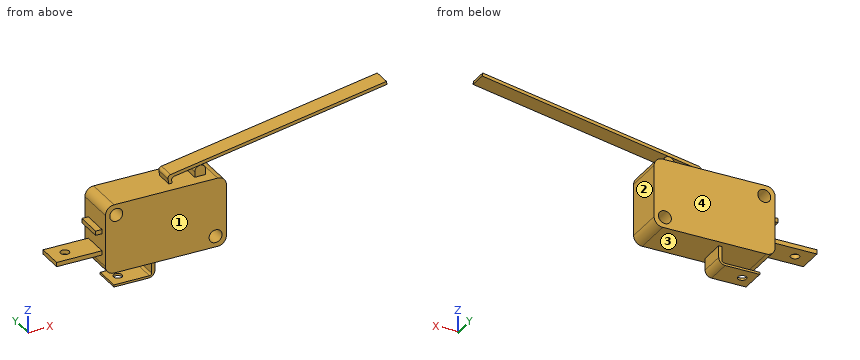
```python
from build123d import *

# Parameters (mm, degrees)
F0_R           = 1.5
F1_DEPTH       = 4.5
F0_W           = 1.5
F0_H           = 1
F0_W_2         = 10.5
F2_DEPTH       = 3
F3_DEPTH       = 2
F4_DEPTH       = 4.5
F5_DEPTH       = 3
F6_DEPTH       = 2
F9_D           = 2
F9_DEPTH       = 1
F9_TIP         = 0.600860619
F9_ON_F8_D     = 2
F9_ON_F8_DEPTH = 1
F9_ON_F8_TIP   = 0.600860619


with BuildPart() as f1:
    # F0 (on Front) → F1 (new body)
    with BuildSketch(Plane.XZ):
        with BuildLine():
            Line((16.1163130835, 15.3639883176), (2.1163130835, 15.3639883176))
            ThreePointArc((2.1163130835, 15.3639883176), (0.7020995211, 14.77820188), (0.1163130835, 13.3639883176))
            Line((0.1163130835, 13.3639883176), (0.1163130835, 9.3639883176))
            Line((0.1163130835, 9.3639883176), (0.1163130835, 8.3639883176))
            Line((0.1163130835, 8.3639883176), (0.1163130835, 4.3639883176))
            Line((0.1163130835, 4.3639883176), (0.1163130835, 3.3639883176))
            Line((0.1163130835, 3.3639883176), (0.1163130835, 1.3639883176))
            ThreePointArc((0.1163130835, 1.3639883176), (0.7020995211, -0.0502252447), (2.1163130835, -0.6360116824))
            Line((2.1163130835, -0.6360116824), (11.6163130835, -0.6360116824))
            Line((11.6163130835, -0.6360116824), (12.3663130835, -0.6360116824))
            Line((12.3663130835, -0.6360116824), (26.1163130835, -0.6360116824))
            ThreePointArc((26.1163130835, -0.6360116824), (27.5305266458, -0.0502252447), (28.1163130835, 1.3639883176))
            Line((28.1163130835, 1.3639883176), (28.1163130835, 13.3639883176))
            ThreePointArc((28.1163130835, 13.3639883176), (27.5305266458, 14.77820188), (26.1163130835, 15.3639883176))
            Line((26.1163130835, 15.3639883176), (24.6163130835, 15.3639883176))
            Line((24.6163130835, 15.3639883176), (23.3663130835, 15.3639883176))
            Line((23.3663130835, 15.3639883176), (22.1163130835, 15.3639883176))
            Line((22.1163130835, 15.3639883176), (16.8778830424, 15.3639883176))
            Line((16.8778830424, 15.3639883176), (16.1163130835, 15.3639883176))
        make_face()
        with Locations((25.6163130835, 1.8639883176)):
            Circle(F0_R, mode=Mode.SUBTRACT)
        with Locations((2.6163130835, 12.8639883176)):
            Circle(F0_R, mode=Mode.SUBTRACT)
    extrude(amount=F1_DEPTH)

    # F0 (on Front) → F2 (join)
    with BuildSketch(Plane.XZ):
        with Locations((-0.6336869165, 8.8639883176)):
            Rectangle(F0_W, F0_H)
        with Locations((-5.1336869165, 3.8639883176)):
            Rectangle(F0_W_2, F0_H)
        with BuildLine():
            Line((12.3663130835, -0.6360116824), (11.6163130835, -0.6360116824))
            Line((11.6163130835, -0.6360116824), (11.6163130835, -3.8694406524))
            ThreePointArc((11.6163130835, -3.8694406524), (11.4698664741, -4.222994043), (11.1163130835, -4.3694406524))
            Line((11.1163130835, -4.3694406524), (2.8663130835, -4.3694406524))
            Line((2.8663130835, -4.3694406524), (2.8663130835, -4.8694406524))
            Line((2.8663130835, -4.8694406524), (10.8663130835, -4.8694406524))
            ThreePointArc((10.8663130835, -4.8694406524), (11.9269732552, -4.4301008242), (12.3663130835, -3.3694406524))
            Line((12.3663130835, -3.3694406524), (12.3663130835, -0.6360116824))
        make_face()
    extrude(amount=F2_DEPTH)

    # F0 (on Front) → F3 (join)
    with BuildSketch(Plane.XZ):
        with BuildLine():
            Line((15.8992528614, 16.5949980089), (16.1163130835, 15.3639883176))
            Line((16.1163130835, 15.3639883176), (16.8778830424, 15.3639883176))
            Line((16.8778830424, 15.3639883176), (16.7680948094, 15.9866283274))
            ThreePointArc((16.7680948094, 15.9866283274), (16.8923365909, 16.5470467879), (17.3764644909, 16.8554702754))
            Line((17.3764644909, 16.8554702754), (66.6168521415, 25.5378791587))
            Line((66.6168521415, 25.5378791587), (66.4866160083, 26.2764849735))
            Line((66.4866160083, 26.2764849735), (16.5076225429, 17.4638399569))
            ThreePointArc((16.5076225429, 17.4638399569), (16.0234946429, 17.1554164694), (15.8992528614, 16.5949980089))
        make_face()
        with BuildLine():
            ThreePointArc((24.6163130835, 16.6139883176), (24.25019656, 15.7301048411), (23.3663130835, 15.3639883176))
            Line((23.3663130835, 15.3639883176), (24.6163130835, 15.3639883176))
            Line((24.6163130835, 15.3639883176), (24.6163130835, 16.6139883176))
        make_face()
        with BuildLine():
            Line((22.1163130835, 16.6139883176), (22.1163130835, 15.3639883176))
            Line((22.1163130835, 15.3639883176), (23.3663130835, 15.3639883176))
            ThreePointArc((23.3663130835, 15.3639883176), (22.482429607, 15.7301048411), (22.1163130835, 16.6139883176))
        make_face()
        with BuildLine():
            ThreePointArc((22.1163130835, 16.6139883176), (22.482429607, 15.7301048411), (23.3663130835, 15.3639883176))
            ThreePointArc((23.3663130835, 15.3639883176), (24.25019656, 15.7301048411), (24.6163130835, 16.6139883176))
            Line((24.6163130835, 16.6139883176), (22.1163130835, 16.6139883176))
        make_face()
        with BuildLine():
            ThreePointArc((24.6163130835, 16.6139883176), (23.3663130835, 17.8639883176), (22.1163130835, 16.6139883176))
            Line((22.1163130835, 16.6139883176), (24.6163130835, 16.6139883176))
        make_face()
    extrude(amount=F3_DEPTH)

    # F0 (on Front) → F4 (join)
    with BuildSketch(Plane.XZ):
        with BuildLine():
            Line((16.1163130835, 15.3639883176), (2.1163130835, 15.3639883176))
            ThreePointArc((2.1163130835, 15.3639883176), (0.7020995211, 14.77820188), (0.1163130835, 13.3639883176))
            Line((0.1163130835, 13.3639883176), (0.1163130835, 9.3639883176))
            Line((0.1163130835, 9.3639883176), (0.1163130835, 8.3639883176))
            Line((0.1163130835, 8.3639883176), (0.1163130835, 4.3639883176))
            Line((0.1163130835, 4.3639883176), (0.1163130835, 3.3639883176))
            Line((0.1163130835, 3.3639883176), (0.1163130835, 1.3639883176))
            ThreePointArc((0.1163130835, 1.3639883176), (0.7020995211, -0.0502252447), (2.1163130835, -0.6360116824))
            Line((2.1163130835, -0.6360116824), (11.6163130835, -0.6360116824))
            Line((11.6163130835, -0.6360116824), (12.3663130835, -0.6360116824))
            Line((12.3663130835, -0.6360116824), (26.1163130835, -0.6360116824))
            ThreePointArc((26.1163130835, -0.6360116824), (27.5305266458, -0.0502252447), (28.1163130835, 1.3639883176))
            Line((28.1163130835, 1.3639883176), (28.1163130835, 13.3639883176))
            ThreePointArc((28.1163130835, 13.3639883176), (27.5305266458, 14.77820188), (26.1163130835, 15.3639883176))
            Line((26.1163130835, 15.3639883176), (24.6163130835, 15.3639883176))
            Line((24.6163130835, 15.3639883176), (23.3663130835, 15.3639883176))
            Line((23.3663130835, 15.3639883176), (22.1163130835, 15.3639883176))
            Line((22.1163130835, 15.3639883176), (16.8778830424, 15.3639883176))
            Line((16.8778830424, 15.3639883176), (16.1163130835, 15.3639883176))
        make_face()
        with Locations((25.6163130835, 1.8639883176)):
            Circle(F0_R, mode=Mode.SUBTRACT)
        with Locations((2.6163130835, 12.8639883176)):
            Circle(F0_R, mode=Mode.SUBTRACT)
    extrude(amount=-F4_DEPTH)

    # F0 (on Front) → F5 (join)
    with BuildSketch(Plane.XZ):
        with Locations((-0.6336869165, 8.8639883176)):
            Rectangle(F0_W, F0_H)
        with Locations((-5.1336869165, 3.8639883176)):
            Rectangle(F0_W_2, F0_H)
        with BuildLine():
            Line((12.3663130835, -0.6360116824), (11.6163130835, -0.6360116824))
            Line((11.6163130835, -0.6360116824), (11.6163130835, -3.8694406524))
            ThreePointArc((11.6163130835, -3.8694406524), (11.4698664741, -4.222994043), (11.1163130835, -4.3694406524))
            Line((11.1163130835, -4.3694406524), (2.8663130835, -4.3694406524))
            Line((2.8663130835, -4.3694406524), (2.8663130835, -4.8694406524))
            Line((2.8663130835, -4.8694406524), (10.8663130835, -4.8694406524))
            ThreePointArc((10.8663130835, -4.8694406524), (11.9269732552, -4.4301008242), (12.3663130835, -3.3694406524))
            Line((12.3663130835, -3.3694406524), (12.3663130835, -0.6360116824))
        make_face()
    extrude(amount=-F5_DEPTH)

    # F0 (on Front) → F6 (join)
    with BuildSketch(Plane.XZ):
        with BuildLine():
            ThreePointArc((24.6163130835, 16.6139883176), (23.3663130835, 17.8639883176), (22.1163130835, 16.6139883176))
            Line((22.1163130835, 16.6139883176), (24.6163130835, 16.6139883176))
        make_face()
        with BuildLine():
            ThreePointArc((22.1163130835, 16.6139883176), (22.482429607, 15.7301048411), (23.3663130835, 15.3639883176))
            ThreePointArc((23.3663130835, 15.3639883176), (24.25019656, 15.7301048411), (24.6163130835, 16.6139883176))
            Line((24.6163130835, 16.6139883176), (22.1163130835, 16.6139883176))
        make_face()
        with BuildLine():
            ThreePointArc((24.6163130835, 16.6139883176), (24.25019656, 15.7301048411), (23.3663130835, 15.3639883176))
            Line((23.3663130835, 15.3639883176), (24.6163130835, 15.3639883176))
            Line((24.6163130835, 15.3639883176), (24.6163130835, 16.6139883176))
        make_face()
        with BuildLine():
            Line((22.1163130835, 16.6139883176), (22.1163130835, 15.3639883176))
            Line((22.1163130835, 15.3639883176), (23.3663130835, 15.3639883176))
            ThreePointArc((23.3663130835, 15.3639883176), (22.482429607, 15.7301048411), (22.1163130835, 16.6139883176))
        make_face()
        with BuildLine():
            Line((15.8992528614, 16.5949980089), (16.1163130835, 15.3639883176))
            Line((16.1163130835, 15.3639883176), (16.8778830424, 15.3639883176))
            Line((16.8778830424, 15.3639883176), (16.7680948094, 15.9866283274))
            ThreePointArc((16.7680948094, 15.9866283274), (16.8923365909, 16.5470467879), (17.3764644909, 16.8554702754))
            Line((17.3764644909, 16.8554702754), (66.6168521415, 25.5378791587))
            Line((66.6168521415, 25.5378791587), (66.4866160083, 26.2764849735))
            Line((66.4866160083, 26.2764849735), (16.5076225429, 17.4638399569))
            ThreePointArc((16.5076225429, 17.4638399569), (16.0234946429, 17.1554164694), (15.8992528614, 16.5949980089))
        make_face()
    extrude(amount=-F6_DEPTH)

    # F9
    with Locations(Plane(origin=(0, 0, -4.8694406524), x_dir=(1, 0, 0), z_dir=(0, 0, -1))):
        with Locations((5.3663130835, 0)):
            Hole(F9_D / 2, depth=F9_DEPTH)
            with Locations((0, 0, -(F9_DEPTH + F9_TIP / 2))):  # 118° drill point
                Cone(0, F9_D / 2, F9_TIP, mode=Mode.SUBTRACT)

    # F9 on F8
    with Locations(Plane(origin=(0, 0, 3.3639883176), x_dir=(1, 0, 0), z_dir=(0, 0, -1))):
        with Locations((-6.8836869165, 0)):
            Hole(F9_ON_F8_D / 2, depth=F9_ON_F8_DEPTH)
            with Locations((0, 0, -(F9_ON_F8_DEPTH + F9_ON_F8_TIP / 2))):  # 118° drill point
                Cone(0, F9_ON_F8_D / 2, F9_ON_F8_TIP, mode=Mode.SUBTRACT)


solid = f1.part
```
Check sheet for the modelled part. Datum: model origin and axes. Units: mm. Face numbers are marked on the shaded views. A direction names the side the tool comes from. Give positions to 0.01 mm unless a question says otherwise; leave off trailing zeros. Order: outer loops, then holes, each group sorted by start corner. A loop starts at its lowest first (then second) coordinate and runs counter-clockwise, first axis right, second up. Notation, with made-up numbers: (62.25, 26.5) -> (81.25, 26.5) arc R34 ccw to (81.25, 62.5) -> close; hole circle Ø4 at (1, 84). An arc over 180 degrees is marked (long way). Use CSV: the item, a comma, the result in double quotes. Start each with the question number.
1) Go/stop test with flat-tipped pins: P1, Ø5, axis at y = 1, z = 12, coming from the +X side; P2, Ø2, axis at x = 23.5, z = 17, coming from the +Y side; P3, Ø0.8, axis at x = 23.5, z = 16.5, coming from the -Y side; P4, Ø5, axis at x = 32.5, z = 16, coming from the -Y side. Record where each tip stops, or that it passes through.
2) Sectioned sample at C-C, the plane x = 19. Record the boundary of the cut face in (y, z).
3) Sectioned sample at B-B, the plane y = 0. Give the number of separate pieces and of enclosed holes in the cut face, plus the area to 3 significant figures.
4) Set-up check for the marked faces 1 and 2: record each of +Z, -Z, +X, -X, +Y, -Y from which the full face is reachable in a straight line by a thin tool's end or side.
5) Sectioned sample at A-A, the plane x = 8. Record the boundary of the cut face in (y, z).
6) Sectioned sample at D-D, the plane x = 47.5. Record the boundary of the cut face in (y, z), plus the area to 3 significant figures.
7) Material ranges on line 1 (Z direction, x = 0, y = 1); line 2 (X direction, y = -3, z = 6); line 3 (Z direction, x = 7, y = -2.5), recorded low to high. Write a range as from..to.
8) Mould release check, pull along Z, two halves, no side actions. Record for the marked faces 3 and 4: released by +Z, released by -Z, zero draft, split by the parting line, or undercut.
Recorded:
1,P1,"x = 28.12"
1,P2,"y = 2"
1,P3,"y = -2"
1,P4,"through"
2,outline,"(-4.5, -0.64) -> (4.5, -0.64) -> (4.5, 15.36) -> (-4.5, 15.36) -> close; (-2, 17.14) -> (2, 17.14) -> (2, 17.9) -> (-2, 17.9) -> close"
3,separate pieces,"3"
3,enclosed holes,"2"
3,area,"492 mm2"
4,face 1,"+Z, -Z, +X, -X, -Y"
4,face 2,"-Z, +X, +Y, -Y"
5,outline,"(-4.5, -0.64) -> (4.5, -0.64) -> (4.5, 15.36) -> (-4.5, 15.36) -> close; (-3, -4.87) -> (3, -4.87) -> (3, -4.37) -> (-3, -4.37) -> close"
6,outline,"(-2, 22.17) -> (2, 22.17) -> (2, 22.93) -> (-2, 22.93) -> close"
6,area,"3.05 mm2"
7,line 1,"3.36..4.36, 8.36..9.36"
7,line 2,"0.12..28.12"
7,line 3,"-4.87..-4.37, -0.64..15.36"
8,face 3,"undercut"
8,face 4,"zero draft"
